from build123d import *


with BuildPart() as part:
    # Sketch1 → Base-Revolve (revolve)
    with BuildSketch(Plane.XY, mode=Mode.PRIVATE) as base_revolve_sk:
        Polygon((0, 12.7), (0, 25.4), (25.4, 25.4), (25.4, 38.1), (38.1, 38.1), (38.1, 34.925), (44.45, 34.925), (44.45, 38.1), (57.15, 38.1), (57.15, 25.4), (82.55, 25.4), (82.55, 12.7), align=None)
    revolve(base_revolve_sk.sketch.rotate(Axis((0, 0, 0), (1, 0, 0)), 90), axis=Axis((0, 0, 0), (1, 0, 0)))


solid = part.part
Verification items for the finished model (mm, model axes). A direction names the side the tool comes from. Coordinates: 2 decimals unless noted, no trailing zeros. Write each loop counter-clockwise with the first axis right and the second up, starting at its lowest first coordinate (ties: lowest second). Pieces come first, ordered by that corner, then holes. Notation, with made-up numbers: M -24.75,-30 L 24.25,-30 A20 ccw 24.25,-20 Z; hole C -16,25 d4. An arc over 180 degrees is marked long. Use CSV: the item, a comma, the result in double quotes.
Q1. Set-up check for faces 1 (the cylindrical face through (70.028, 15.456, -20.157)), 2 (the flat face through (44.45, 31, -17)), 3 (the flat face through (25.4, 8, -25)), 4 (the cylindrical face through (40.7, 7.7, -10.1)), 5 (the flat face through (0, -12, -5)): record each of +Z, -Z, +X, -X, +Y, -Y from which the full face is reachable in a straight line by a thin tool's end or side.
Computed values:
face 1,"+X"
face 2,"none"
face 3,"-X"
face 4,"+X, -X"
face 5,"+Z, -Z, -X, +Y, -Y"
Q2. Section check A-A, the plane z = 0. Enter the section's corners in (x, y) (3 decimals).
Computed values:
outline,"M 0,-25.4 L 25.4,-25.4 L 25.4,-38.1 L 38.1,-38.1 L 38.1,-34.925 L 44.45,-34.925 L 44.45,-38.1 L 57.15,-38.1 L 57.15,-25.4 L 82.55,-25.4 L 82.55,-12.7 L 0,-12.7 Z; M 0,12.7 L 82.55,12.7 L 82.55,25.4 L 57.15,25.4 L 57.15,38.1 L 44.45,38.1 L 44.45,34.925 L 38.1,34.925 L 38.1,38.1 L 25.4,38.1 L 25.4,25.4 L 0,25.4 Z"
Q3. Mould release check, pull along X, two halves, no side actions. Record for faces 6 (the cylindrical face through (12.878, 15.456, -20.157)), 7 (the flat face through (38.1, 31, 17)), 8 (the flat face through (57.15, 8, 25)), 9 (the cylindrical face through (41.319, 34.094, -7.571)): pulls with the +X half, pulls with the -X half, needs draft (parallel to the pull), parting line crosses it, or undercut.
Computed values:
face 6,"needs draft"
face 7,"undercut"
face 8,"pulls with the +X half"
face 9,"undercut"
Q4. Thickness scan on line 1 along Y through (x, z) = (54.5, 0); line 2 along Y through (x, z) = (44, 0) (3 decimals); line 3 along X through (y, z) = (-21, -30). Record the ranges inside material, lowest first. Write a range as [from, to].
Computed values:
line 1,"[-38.1, -12.7], [12.7, 38.1]"
line 2,"[-34.925, -12.7], [12.7, 34.925]"
line 3,"[25.4, 38.1], [44.45, 57.15]"
Q5. Go/stop test with flat-tipped pins: P1, Ø1, axis at x = 56.5, z = 11, coming from the -Y side; P2, Ø5, axis at y = 30, z = -4.5, coming from the -X side; P3, Ø4, axis at x = 34.5, y = 18, coming from the +Z side. Record where each tip stops, or that it passes through.
Computed values:
P1,"y = -36.62"
P2,"x = 25.4"
P3,"z = 34.58"
Q6. Section check D-D, the plane z = 19.5. Enter the section's corners in (x, y).
Computed values:
outline,"M 0,-16.28 L 25.4,-16.28 L 25.4,-32.73 L 38.1,-32.73 L 38.1,-28.97 L 44.45,-28.97 L 44.45,-32.73 L 57.15,-32.73 L 57.15,-16.28 L 82.55,-16.28 L 82.55,16.28 L 57.15,16.28 L 57.15,32.73 L 44.45,32.73 L 44.45,28.97 L 38.1,28.97 L 38.1,32.73 L 25.4,32.73 L 25.4,16.28 L 0,16.28 Z"
Q7. Section check C-C, the plane x = 73. Enter the section's corners in (y, z), and give its area (3 significant figures).
Computed values:
outline,"C 0,0 d50.8; hole C 0,0 d25.4"
area,"1,520 mm²"
